Could you check a few things on this drawing? It's one solid part, dimensions in mm from its lowest x, y, z. A direction names the side the tool comes from. Round coordinates to 2 decimals unless told otherwise and drop trailing zeros. Write each loop counter-clockwise with the first axis right and the second up, starting at its lowest first coordinate (ties: lowest second). Pieces come first, ordered by that corner, then holes. Notation, with made-up numbers: (34, -23.75) -> (44, -23.75) arc R18 cw to (44, -7.75) -> close; hole circle Ø2 at (55.25, 1). An arc over 180 degrees is marked (long way). Answer in a Markdown table with one row per item.
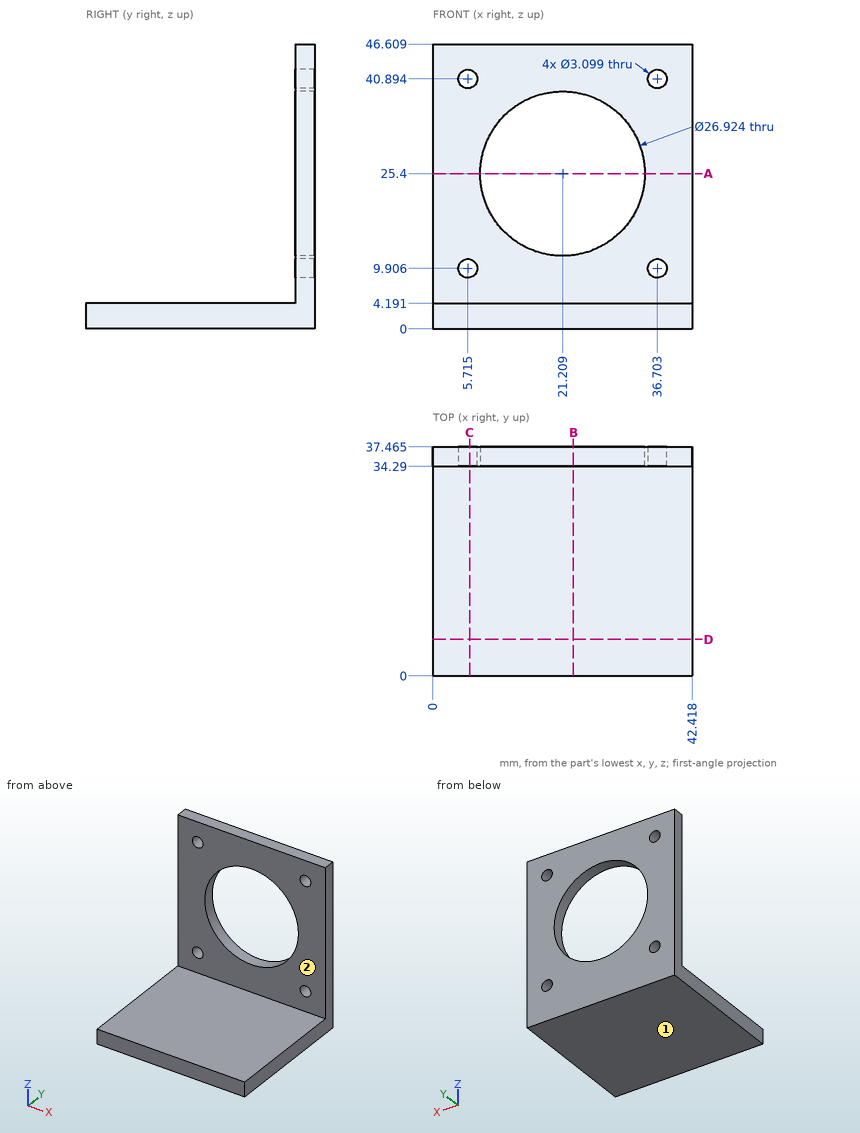
1) Imagine slicing it at A-A, the plane z = 25.4. Please give me the cut outline in (x, y) (3 decimals).
Findings:
| item | result |
|---|---|
| outline | (0, 34.29) -> (7.747, 34.29) -> (7.747, 37.465) -> (0, 37.465) -> close; (34.671, 34.29) -> (42.418, 34.29) -> (42.418, 37.465) -> (34.671, 37.465) -> close |
2) Imagine slicing it at D-D, the plane y = 6. Please give me the cut outline in (x, z), plus the area to 3 significant figures.
Findings:
| item | result |
|---|---|
| outline | (0, 0) -> (42.42, 0) -> (42.42, 4.19) -> (0, 4.19) -> close |
| area | 178 mm^2 |
3) Imagine slicing it at B-B, the plane x = 23. Please give me the cut outline in (y, z) (1 decimal), plus the area to 3 significant figures.
Findings:
| item | result |
|---|---|
| outline | (0, 0) -> (37.5, 0) -> (37.5, 12.1) -> (34.3, 12.1) -> (34.3, 4.2) -> (0, 4.2) -> close; (34.3, 38.7) -> (37.5, 38.7) -> (37.5, 46.6) -> (34.3, 46.6) -> close |
| area | 207 mm^2 |
4) For pin 1 (6 mm diameter, centred on y = 22, z = 8, fed in from -X); pin 2 (1.5 mm diameter, centred on x = 27, y = 5, fed in from +Z); pin 3 (12 mm diameter, centred on x = 27.5, z = 40.5, fed in from -Y), each with a flat end and sliding along its axis, tell me the tip position at first contact or that it passes through.
Findings:
| item | result |
|---|---|
| pin 1 | passes through |
| pin 2 | stops at z = 4.19 |
| pin 3 | stops at y = 34.29 |
5) Please list where these lines run through material, in increasing order: line 1 (X direction, y = 36, z = 25) (3 decimals); line 2 (Z direction, x = 17, y = 32); line 3 (Y direction, x = 2.5, z = 5.5) (3 decimals).
Findings:
| item | result |
|---|---|
| line 1 | x = 0 to 7.753, 34.665 to 42.418 |
| line 2 | z = 0 to 4.19 |
| line 3 | y = 34.29 to 37.465 |
6) For the marked faces 1 and 2, which set-ups out of +Z, -Z, +X, -X, +Y, -Y let a thin tool reach every point of the face, with its end or its side?
Findings:
| item | result |
|---|---|
| face 1 | -Z, +X, -X, +Y, -Y |
| face 2 | +Z, +X, -X, -Y |
7) Imagine slicing it at C-C, the plane x = 6. Please give me the cut outline in (y, z) (3 decimals), plus the area to 3 significant figures.
Findings:
| item | result |
|---|---|
| outline | (0, 0) -> (37.465, 0) -> (37.465, 8.383) -> (34.29, 8.383) -> (34.29, 4.191) -> (0, 4.191) -> close; (34.29, 11.429) -> (37.465, 11.429) -> (37.465, 39.371) -> (34.29, 39.371) -> close; (34.29, 42.417) -> (37.465, 42.417) -> (37.465, 46.609) -> (34.29, 46.609) -> close |
| area | 272 mm^2 |
